For this review, take the finished solid that the model builds, in its own axes (mm). Face numbers are marked on the shaded views. A direction names the side the tool comes from. Give positions to 0.01 mm unless a question says otherwise; leave off trailing zeros. Write each loop counter-clockwise with the first axis right and the second up, starting at its lowest first coordinate (ties: lowest second). Pieces come first, ordered by that corner, then holes.
1) Machinability: for the marked faces 1, 2 and 3, which of the approach directions +Z, -Z, +X, -X, +Y, -Y give a long, thin tool a straight path to every point of the face, cutting with its end or side? Answer none if there is none.
2) Draft analysis for pull direction Z (two halves, no side actions). For the marked faces 4, 5, 6 and 7, state which applies: pulls with the +Z half, pulls with the -Z half, needs draft (parallel to the pull), parting line crosses it, or undercut.
3) We need section B-B on z = 30. Give the boundary of the cut face in (x, y).
4) For P1, Ø5, axis at y = 6, z = 2, coming from the +X side; P2, Ø12, axis at x = 5.5, z = 30.5, coming from the +Y side; P3, Ø6, axis at y = 6.5, z = 1.5, coming from the +X side; P4, Ø3.5, axis at x = -49, z = -16, coming from the -Y side, all flat-tipped, find the tip position at first contact; note any pin that passes through.
5) Wall thickness on line 1 along X through (y, z) = (6, -16); line 2 along Z through (x, y) = (-29.5, 6.75); line 3 along Z through (x, y) = (-28, 6.5): over which ranges is each line inside the solid? List them lowest first.
6) We need section A-A on x = -25. Give the boundary of the cut face in (y, z).
7) We need section D-D on x = -49. Give the boundary of the cut face in (y, z), and give its area (3 significant figures).
8) We need section C-C on x = 41. Give the boundary of the cut face in (y, z).
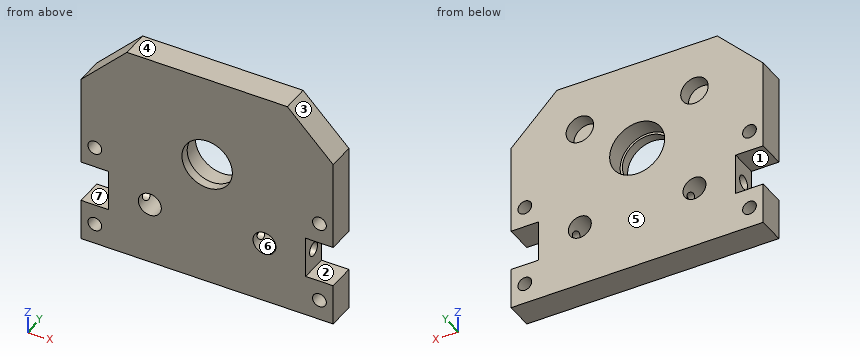
from build123d import *

# Parameters (mm, degrees)
SKETCH1_W           = 66
SKETCH1_H           = 95
SKETCH1_R           = 11
BOSS_EXTRUDE1_DEPTH = 12
BOSS_EXTRUDE3_DEPTH = 12
SKETCH4_R           = 12
CUT_EXTRUDE1_DEPTH  = 8
SKETCH6_R           = 6
CUT_EXTRUDE2_DEPTH  = 6
CHAMFER1_SIZE       = 20
CUT_EXTRUDE3_REACH  = 91.828
SKETCH7_R           = 3
SKETCH7_R_2         = 5
SKETCH9_R           = 3
CUT_EXTRUDE5_DEPTH  = 25


with BuildPart() as part:
    # Sketch1 → Boss-Extrude1 (new body)
    with BuildSketch(Plane(origin=(0, 0, 0), x_dir=(1, 0, 0), z_dir=(0, 1, 0))):
        with Locations((0, -22.5)):
            Rectangle(SKETCH1_W, SKETCH1_H)
        with Locations(Location((0, -30, 0), (0, 0, 270))):
            Circle(SKETCH1_R, mode=Mode.SUBTRACT)
    extrude(amount=BOSS_EXTRUDE1_DEPTH)

    # Sketch3 → Boss-Extrude3 (add)
    with BuildSketch(Plane(origin=(0, 12, 0), x_dir=(1, 0, 0), z_dir=(0, 1, 0))):
        Polygon((55, 7), (43, 7), (43, -11), (55, -11), (55, -70), (33, -70), (33, 25), (55, 25), align=None)
    boss_extrude3 = extrude(amount=-BOSS_EXTRUDE3_DEPTH)

    # Mirror1: Boss-Extrude3 across plane
    add(boss_extrude3.mirror(Plane(origin=(0, 0, 0), x_dir=(0, 0, 1), z_dir=(1, 0, 0))))

    # Sketch4 → Cut-Extrude1 (cut)
    with BuildSketch(Plane(origin=(0, 12, 0), x_dir=(1, 0, 0), z_dir=(0, 1, 0))):
        with Locations(Location((0, -30, 0), (0, 0, 270))):
            Circle(SKETCH4_R)
    extrude(amount=-CUT_EXTRUDE1_DEPTH, mode=Mode.SUBTRACT)

    # Sketch6 → Cut-Extrude2 (cut)
    with BuildSketch(Plane(origin=(0, 12, 0), x_dir=(1, 0, 0), z_dir=(0, 1, 0))):
        with Locations(Location((-25, -48, 0), (0, 0, 270))):
            Circle(SKETCH6_R)
        with Locations(Location((25, -48, 0), (0, 0, 270))):
            Circle(SKETCH6_R)
    extrude(amount=-CUT_EXTRUDE2_DEPTH, mode=Mode.SUBTRACT)

    # Chamfer1
    chamfer1_edges = [part.edges().sort_by_distance(p)[0] for p in [
        (55, 6, 70),
        (-55, 6, 70),
    ]]
    chamfer(chamfer1_edges, length=CHAMFER1_SIZE)

    # Sketch7 → Cut-Extrude3 (cut, up to next)
    with BuildSketch(Plane(origin=(0, 12, 0), x_dir=(1, 0, 0), z_dir=(0, 1, 0)), mode=Mode.PRIVATE) as cut_extrude3_sk1:
        with Locations(Location((-49, 16, 0), (0, 0, 270))):
            Circle(SKETCH7_R)
    cut_extrude3_tool1 = extrude(cut_extrude3_sk1.sketch, amount=-CUT_EXTRUDE3_REACH, mode=Mode.PRIVATE) & part.part
    # Sketch7 → Cut-Extrude3 (cut, up to next)
    with BuildSketch(Plane(origin=(0, 12, 0), x_dir=(1, 0, 0), z_dir=(0, 1, 0)), mode=Mode.PRIVATE) as cut_extrude3_sk2:
        with Locations(Location((-49, -20, 0), (0, 0, 270))):
            Circle(SKETCH7_R)
    cut_extrude3_tool2 = extrude(cut_extrude3_sk2.sketch, amount=-CUT_EXTRUDE3_REACH, mode=Mode.PRIVATE) & part.part
    # Sketch7 → Cut-Extrude3 (cut, up to next)
    with BuildSketch(Plane(origin=(0, 12, 0), x_dir=(1, 0, 0), z_dir=(0, 1, 0)), mode=Mode.PRIVATE) as cut_extrude3_sk3:
        with Locations(Location((-25, -2, 0), (0, 0, 270))):
            Circle(SKETCH7_R_2)
    cut_extrude3_tool3 = extrude(cut_extrude3_sk3.sketch, amount=-CUT_EXTRUDE3_REACH, mode=Mode.PRIVATE) & part.part
    cut_extrude3_1 = cut_extrude3_tool1.solids().sort_by_distance((-49, 12, -16))[0]
    add(cut_extrude3_1, mode=Mode.SUBTRACT)
    cut_extrude3_2 = cut_extrude3_tool2.solids().sort_by_distance((-49, 12, 20))[0]
    add(cut_extrude3_2, mode=Mode.SUBTRACT)
    cut_extrude3_3 = cut_extrude3_tool3.solids().sort_by_distance((-25, 12, 2))[0]
    add(cut_extrude3_3, mode=Mode.SUBTRACT)
    cut_extrude3 = cut_extrude3_1 + cut_extrude3_2 + cut_extrude3_3  # Cut-Extrude3 as one shape, for the pattern or mirror that repeats it

    # Sketch9 → Cut-Extrude5 (cut)
    with BuildSketch(Plane.ZY.offset(43)):
        with Locations((2, 6)):
            Circle(SKETCH9_R)
    cut_extrude5 = extrude(amount=-CUT_EXTRUDE5_DEPTH, mode=Mode.SUBTRACT)

    # Mirror2: Cut-Extrude3, Cut-Extrude5 across plane
    add(cut_extrude3.mirror(Plane(origin=(0, 0, 0), x_dir=(0, 0, 1), z_dir=(1, 0, 0))), mode=Mode.SUBTRACT)
    add(cut_extrude5.mirror(Plane(origin=(0, 0, 0), x_dir=(0, 0, 1), z_dir=(1, 0, 0))), mode=Mode.SUBTRACT)


solid = part.part
Results list:
1. face 1: -X, +Y, -Y
1. face 2: +X, +Y, -Y
1. face 3: +Z, +X, +Y, -Y
2. face 4: pulls with the +Z half
2. face 5: needs draft
2. face 6: undercut
2. face 7: undercut
3. outline: (-55, 0) - (-11, 0) - (-11, 4) - (-12, 4) - (-12, 12) - (-55, 12) - close; (11, 0) - (55, 0) - (55, 12) - (12, 12) - (12, 4) - (11, 4) - close
4. P1: stops at x = 18
4. P2: stops at y = 4
4. P3: stops at x = 43
4. P4: passes through
5. line 1: x = -55 to -52, -46 to 46, 52 to 55
5. line 2: z = -25 to -0.9, 4.9 to 44.03, 51.97 to 70
5. line 3: z = -25 to -2, 6 to 42.8, 53.2 to 70
6. outline: (0, -25) - (12, -25) - (12, -3) - (0, -3) - close; (0, 7) - (12, 7) - (12, 42) - (6, 42) - (6, 54) - (12, 54) - (12, 70) - (0, 70) - close
7. outline: (0, -25) - (12, -25) - (12, -19) - (0, -19) - close; (0, -13) - (12, -13) - (12, -7) - (0, -7) - close; (0, 11) - (12, 11) - (12, 17) - (0, 17) - close; (0, 23) - (12, 23) - (12, 56) - (0, 56) - close
7. area: 612 mm2
8. outline: (0, -25) - (12, -25) - (12, 64) - (0, 64) - close; hole circle Ø6 at (6, 2)
